Here's how the part is built. I have some questions about the finished solid (model axes, mm). Coordinates: 2 decimals unless noted, no trailing zeros. Order: outer loops, then holes, each group sorted by start corner. A loop starts at its lowest first (then second) coordinate and runs counter-clockwise, first axis right, second up. Notation, with made-up numbers: (60, 73.25) - (88, 73.25) arc R27 ccw to (88, 89.25) - close; hole circle Ø11 at (36, 36.5). An arc over 180 degrees is marked (long way). Answer in a Markdown table with one row per item. Add a question column.
Item 1: I want a section at D-D (y = 41.5). Please give me the cut outline in (x, z), plus the area to 3 significant figures.
Item 2: Thinking about a two-plate mould opening in X: for faces 1 (the flat face through (11.22, 19.31, 2.54)), 2 (the flat face through (-1, -10, 0)), which applies, +X half, -X half, draft (parallel to the pull), parting line (faces both ways), or undercut?
Item 3: I want a section at B-B (y = -46.3). Please give me the cut outline in (x, z).
Item 4: If I drill on line 1 along Y through (x, z) = (-39, 0.75); line 2 along X through (y, z) = (19, 1.6); line 3 along Y through (x, z) = (-44, 0.4), over which ranges is the centre line in solid material (lowest first)? Write a range as from..to.
Item 5: I want a section at A-A (x = 0). Please give me the cut outline in (y, z).
Item 6: I want a section at C-C (z = 1.45). Count the separate pieces of the cut face and the enclosed holes in it, plus the area to 3 significant figures.
Item 7: Will these pins go through, and if not, where does the flat tip stop? pin 1 Ø1.8 at (y, z) = (-2.5, 2) entering from +X; pin 2 Ø1.8 at (x, z) = (22, 3.5) entering from +Y; pin 3 Ø2 at (y, z) = (35.5, 1) entering from +X.
```python
from build123d import *

# Parameters (mm, degrees)
BOSS_EXTRU_1_OUTLINE_R   = 50
BOSS_EXTRU_1_OUTLINE_W   = 5
BOSS_EXTRU_1_OUTLINE_H   = 5
BOSS_EXTRU_1_OUTLINE_R_2 = 2.05
BOSS_EXTRU_1_OUTLINE_R_3 = 1.5
BOSS_EXTRU_1_DEPTH       = 5
SKETCH3_W                = 1
SKETCH3_H                = 8
CUT_EXTRUDE2_DEPTH       = 10


# Read off the part's stored shape, not the designer's step: Boss.-Extru.1
with BuildPart() as part:
    # Boss.-Extru.1 outline → Boss.-Extru.1 (new body)
    with BuildSketch(Plane.XY):
        Circle(BOSS_EXTRU_1_OUTLINE_R)
        Polygon((-37.262039705, -33.060254038), (-39.762039705, -28.730127019), (-35.431912686, -26.230127019), (-32.931912686, -30.560254038), align=None, mode=Mode.SUBTRACT)
        with Locations((-7.5, -46.3)):
            Rectangle(BOSS_EXTRU_1_OUTLINE_W, BOSS_EXTRU_1_OUTLINE_H, mode=Mode.SUBTRACT)
        with Locations((-16.666666667, -28.867513459)):
            Circle(BOSS_EXTRU_1_OUTLINE_R_2, mode=Mode.SUBTRACT)
        with Locations((-40.096976195, -23.15)):
            Circle(BOSS_EXTRU_1_OUTLINE_R_3, mode=Mode.SUBTRACT)
        Polygon((-42.931912686, -13.239745962), (-40.431912686, -17.569872981), (-44.762039705, -20.069872981), (-47.262039705, -15.739745962), align=None, mode=Mode.SUBTRACT)
        with Locations((0, -46.3)):
            Circle(BOSS_EXTRU_1_OUTLINE_R_3, mode=Mode.SUBTRACT)
        with Locations((7.5, -46.3)):
            Rectangle(BOSS_EXTRU_1_OUTLINE_W, BOSS_EXTRU_1_OUTLINE_H, mode=Mode.SUBTRACT)
        with Locations((16.666666667, -28.867513459)):
            Circle(BOSS_EXTRU_1_OUTLINE_R_2, mode=Mode.SUBTRACT)
        Polygon((32.931912686, -30.560254038), (35.431912686, -26.230127019), (39.762039705, -28.730127019), (37.262039705, -33.060254038), align=None, mode=Mode.SUBTRACT)
        with Locations((40.096976195, -23.15)):
            Circle(BOSS_EXTRU_1_OUTLINE_R_3, mode=Mode.SUBTRACT)
        Polygon((47.262039705, -15.739745962), (44.762039705, -20.069872981), (40.431912686, -17.569872981), (42.931912686, -13.239745962), align=None, mode=Mode.SUBTRACT)
        with Locations((-33.333333333, 0)):
            Circle(BOSS_EXTRU_1_OUTLINE_R_2, mode=Mode.SUBTRACT)
        Polygon((-47.262039705, 15.739745962), (-44.762039705, 20.069872981), (-40.431912686, 17.569872981), (-42.931912686, 13.239745962), align=None, mode=Mode.SUBTRACT)
        with Locations((-40.096976195, 23.15)):
            Circle(BOSS_EXTRU_1_OUTLINE_R_3, mode=Mode.SUBTRACT)
        with Locations((-16.671397032, 9.625235564)):
            Circle(BOSS_EXTRU_1_OUTLINE_R_2, mode=Mode.SUBTRACT)
        Polygon((-32.931912686, 30.560254038), (-35.431912686, 26.230127019), (-39.762039705, 28.730127019), (-37.262039705, 33.060254038), align=None, mode=Mode.SUBTRACT)
        with Locations((-16.666666667, 28.867513459)):
            Circle(BOSS_EXTRU_1_OUTLINE_R_2, mode=Mode.SUBTRACT)
        with Locations((-7.5, 46.3)):
            Rectangle(BOSS_EXTRU_1_OUTLINE_W, BOSS_EXTRU_1_OUTLINE_H, mode=Mode.SUBTRACT)
        Circle(BOSS_EXTRU_1_OUTLINE_R_2, mode=Mode.SUBTRACT)
        with Locations((33.333333333, 0)):
            Circle(BOSS_EXTRU_1_OUTLINE_R_2, mode=Mode.SUBTRACT)
        Polygon((42.931912686, 13.239745962), (40.431912686, 17.569872981), (44.762039705, 20.069872981), (47.262039705, 15.739745962), align=None, mode=Mode.SUBTRACT)
        with Locations((40.096976195, 23.15)):
            Circle(BOSS_EXTRU_1_OUTLINE_R_3, mode=Mode.SUBTRACT)
        with Locations((16.666666667, 28.867513459)):
            Circle(BOSS_EXTRU_1_OUTLINE_R_2, mode=Mode.SUBTRACT)
        with Locations((0, 46.3)):
            Circle(BOSS_EXTRU_1_OUTLINE_R_3, mode=Mode.SUBTRACT)
        with Locations((7.5, 46.3)):
            Rectangle(BOSS_EXTRU_1_OUTLINE_W, BOSS_EXTRU_1_OUTLINE_H, mode=Mode.SUBTRACT)
        Polygon((37.262039705, 33.060254038), (39.762039705, 28.730127019), (35.431912686, 26.230127019), (32.931912686, 30.560254038), align=None, mode=Mode.SUBTRACT)
    extrude(amount=BOSS_EXTRU_1_DEPTH)

    # Sketch3 → Cut-Extrude2 (cut)
    with BuildSketch(Plane.XY.offset(5)):
        with Locations((-22.833333333, 0)):
            Rectangle(SKETCH3_W, SKETCH3_H)
        Polygon((-13.233653965, 23.921361037), (-14.099679369, 23.421361037), (-12.349679369, 20.390272124), (-15.380768282, 18.640272124), (-14.880768282, 17.77424672), (-11.849679369, 19.52424672), (-10.099679369, 16.493157806), (-9.233653965, 16.993157806), (-10.983653965, 20.02424672), (-7.952565052, 21.77424672), (-8.452565052, 22.640272124), (-11.483653965, 20.890272124), align=None)
        Polygon((15.130768282, 18.207259422), (14.630768282, 17.341234018), (7.702565052, 21.341234018), (8.202565052, 22.207259422), align=None)
        Polygon((8.202565052, -22.207259422), (7.702565052, -21.341234018), (14.630768282, -17.341234018), (15.130768282, -18.207259422), align=None)
        Polygon((27.333333333, -0.5), (27.333333333, 0.5), (23.833333333, 0.5), (23.833333333, 4), (22.833333333, 4), (22.833333333, 0.5), (19.333333333, 0.5), (19.333333333, -0.5), (22.833333333, -0.5), (22.833333333, -4), (23.833333333, -4), (23.833333333, -0.5), align=None)
        Polygon((-14.099679369, -23.421361037), (-13.233653965, -23.921361037), (-11.483653965, -20.890272124), (-8.452565052, -22.640272124), (-7.952565052, -21.77424672), (-10.983653965, -20.02424672), (-9.233653965, -16.993157806), (-10.099679369, -16.493157806), (-11.849679369, -19.52424672), (-14.880768282, -17.77424672), (-15.380768282, -18.640272124), (-12.349679369, -20.390272124), align=None)
        Polygon((-7.433012703, 11.874355655), (-5.683012702, 8.843266741), (-8.714101616, 7.093266741), (-8.214101616, 6.227241337), (-5.183012702, 7.977241336), (-3.433012703, 4.946152425), (-2.566987299, 5.446152425), (-4.316987299, 8.477241337), (-1.285898385, 10.227241337), (-1.785898385, 11.093266741), (-4.816987299, 9.343266741), (-6.566987299, 12.374355655), align=None)
        Polygon((-20.834234776, 12.184801987), (-19.940304487, 11.668776346), (-20.102964744, 11.386925384), (-20.996895032, 11.902951025), (-21.517828526, 11.000607275), (-21.800380609, 11.163968654), (-21.279447115, 12.066312404), (-22.173377404, 12.582338045), (-22.010717147, 12.864189006), (-21.116786859, 12.348163365), (-20.596554487, 13.24840375), (-20.314002404, 13.085042371), align=None)
    extrude(amount=-CUT_EXTRUDE2_DEPTH, mode=Mode.SUBTRACT)


solid = part.part
```
Values follow:
| question | item | result |
|---|---|---|
| 1 | outline | (-27.89, 0) - (27.89, 0) - (27.89, 5) - (-27.89, 5) - close |
| 1 | area | 279 mm^2 |
| 2 | face 1 | undercut |
| 2 | face 2 | draft |
| 3 | outline | (-18.88, 0) - (-10, 0) - (-10, 5) - (-18.88, 5) - close; (-5, 0) - (-1.5, 0) - (-1.5, 5) - (-5, 5) - close; (1.5, 0) - (5, 0) - (5, 5) - (1.5, 5) - close; (10, 0) - (18.88, 0) - (18.88, 5) - (10, 5) - close |
| 4 | line 1 | y = -31.29..-30.05, -28.29..-24.17, -22.13..22.13, 24.17..28.29, 30.05..31.29 |
| 4 | line 2 | x = -46.25..-45.38, -42.91..-14.76, -12.76..-11.55, -10.39..11.76, 13.76..42.91, 45.38..46.25 |
| 4 | line 3 | y = -23.75..-19.63, -13.86..13.86, 19.63..23.75 |
| 5 | outline | (-50, 0) - (-47.8, 0) - (-47.8, 5) - (-50, 5) - close; (-44.8, 0) - (-2.05, 0) - (-2.05, 5) - (-44.8, 5) - close; (2.05, 0) - (44.8, 0) - (44.8, 5) - (2.05, 5) - close; (47.8, 0) - (50, 0) - (50, 5) - (47.8, 5) - close |
| 6 | separate pieces | 1 |
| 6 | enclosed holes | 34 |
| 6 | area | 7,320 mm^2 |
| 7 | pin 1 | stops at x = 49.97 |
| 7 | pin 2 | stops at y = 45.33 |
| 7 | pin 3 | stops at x = 36.19 |
